The figure shows three views and two pictorial views of one solid part (mm, origin at its lowest corner). Answer the questions. Give positions to 0.01 mm unless a question says otherwise; leave off trailing zeros. Loops run counter-clockwise (first coordinate to the right, second up) from the corner with the lowest first, then second, coordinate; pieces in that order, holes last. Notation, with made-up numbers: (-9.5, 87) - (16.5, 87) arc R23 cw to (16.5, 124) - close; hole circle Ø5 at (33, -16). An arc over 180 degrees is marked (long way). Write each question's results on one line, items separated by ' | '.
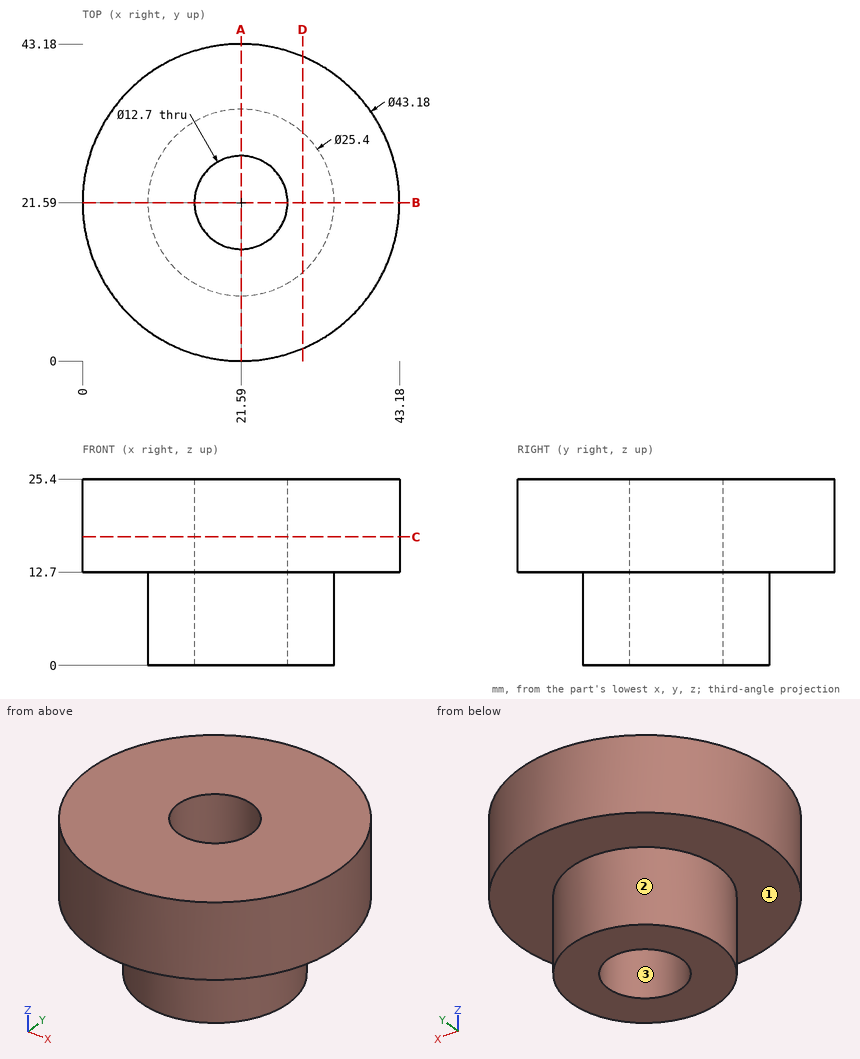
Item 1: A cutting plane is placed at C-C, the plane z = 17.5. Determine the outline of the cut face in (x, y), plus the area to 3 significant figures.
Values found:
outline: circle Ø43.18 at (21.59, 21.59); hole circle Ø12.7 at (21.59, 21.59) | area: 1,340 mm²
Item 2: A cutting plane is placed at A-A, the plane x = 21.59. Determine the outline of the cut face in (y, z), plus the area to 3 significant figures.
Values found:
outline: (0, 12.7) - (8.89, 12.7) - (8.89, 0) - (15.24, 0) - (15.24, 25.4) - (0, 25.4) - close; (27.94, 0) - (34.29, 0) - (34.29, 12.7) - (43.18, 12.7) - (43.18, 25.4) - (27.94, 25.4) - close | area: 548 mm²
Item 3: A cutting plane is placed at D-D, the plane x = 30. Determine the outline of the cut face in (y, z), plus the area to 3 significant figures.
Values found:
outline: (1.71, 12.7) - (12.07, 12.7) - (12.07, 0) - (31.11, 0) - (31.11, 12.7) - (41.47, 12.7) - (41.47, 25.4) - (1.71, 25.4) - close | area: 747 mm²
Item 4: Flat-ended cylindrical pins translate along their axes: P1, Ø7.5, axis at x = 21.59, y = 21.59, coming from the -Z side; P2, Ø2, axis at y = 13.5, z = 17.5, coming from the -X side; P3, Ø1, axis at y = 21.5, z = 10, coming from the -X side; P4, Ø1.5, axis at x = 34, z = 9.5, coming from the +Y side. Find the tip coordinate at first contact, or state that the pin passes through.
Values found:
P1: passes through | P2: stops at x = 1.2 | P3: stops at x = 8.89 | P4: stops at y = 26.62
Item 5: Find the intervals of material crossed by line 1 along Y through (x, z) = (21.59, 7); line 2 along Y through (x, z) = (22, 4.25); line 3 along Z through (x, y) = (6, 18), in increasing order. Write a range as [from, to].
Values found:
line 1: y = [8.89, 15.24], [27.94, 34.29] | line 2: y = [8.9, 15.25], [27.93, 34.28] | line 3: z = [12.7, 25.4]
Item 6: For a pull along Y with two mould halves and no side action, classify the marked faces 1, 2 and 3 as released by +Y, released by -Y, zero draft, split by the parting line, or undercut.
Values found:
face 1: zero draft | face 2: split by the parting line | face 3: undercut
